The model under review builds one solid part; all positions refer to its coordinate system, in mm. Give positions to 0.01 mm unless a question says otherwise; leave off trailing zeros. Order: outer loops, then holes, each group sorted by start corner. A loop starts at its lowest first (then second) coordinate and runs counter-clockwise, first axis right, second up.
```python
from build123d import *

# Parameters (mm, degrees)
F0_R     = 40
F1_DEPTH = 500
F2_R     = 30
F3_R     = 10


with BuildPart() as f1:
    # F0 (on Front) → F1 (new body)
    with BuildSketch(Plane.XZ):
        Circle(F0_R)
    extrude(amount=-F1_DEPTH)

    # F2
    f2_edges = [f1.edges().sort_by_distance(p)[0] for p in [
        (-40, 500, 0),
    ]]
    fillet(f2_edges, radius=F2_R)

    # F3
    f3_edges = [f1.edges().sort_by_distance(p)[0] for p in [
        (-40, 0, 0),
    ]]
    fillet(f3_edges, radius=F3_R)


solid = f1.part
```
Item 1: For line 1 (X direction, y = 229.5, z = 0.5); line 2 (X direction, y = 63, z = -2.5); line 3 (Z direction, x = -1, y = 111.5), list the stretches that pass through material, from the lowest coordinate up.
Values found:
line 1: x = -40 to 40
line 2: x = -39.92 to 39.92
line 3: z = -39.99 to 39.99
Item 2: Take a section at A-A (y = 106). Give the boundary of the cut face in (x, z), and give its area (3 significant figures).
Values found:
outline: circle Ø80 at (0, 0)
area: 5,030 mm2
Item 3: Clearance check with flat-ended pins moving along their axes: pin 1 Ø10 at (x, y) = (-5, 449) entering from +Z; pin 2 Ø12 at (x, y) = (12, 345) entering from -Z; pin 3 Ø12 at (x, y) = (30.5, 186.5) entering from +Z. State where each tip first meets the part, or that it passes through.
Values found:
pin 1: stops at z = 40
pin 2: stops at z = -39.55
pin 3: stops at z = 31.62
